Geometry check sheet. Reference: the model listing, model coordinates, mm. Give positions to 0.01 mm unless a question says otherwise; leave off trailing zeros. Loops run counter-clockwise (first coordinate to the right, second up) from the corner with the lowest first, then second, coordinate; pieces in that order, holes last. Notation, with made-up numbers: (24, 54.5) -> (46, 54.5) arc R25 cw to (46, 81.5) -> close; hole circle Ø1 at (50.25, 37.5). An arc over 180 degrees is marked (long way). Answer in a Markdown table with one row per item. Add a question column.
```python
from build123d import *

# Parameters (mm, degrees)
SKETCH1_R                        = 17.5
BOSS_EXTRUDE1_DEPTH              = 12.5
F_1_2_14_NPSM_TAPPED_HOLE1_D     = 18.9738
F_1_2_14_NPSM_TAPPED_HOLE1_DEPTH = 47.24908
F_1_2_14_NPSM_TAPPED_HOLE1_TIP   = 5.700304607
CHAMFER1_SIZE                    = 5
CHAMFER2_SIZE                    = 2
FILLET1_R                        = 1


with BuildPart() as part:
    # Sketch1 → Boss-Extrude1 (new body, symmetric)
    with BuildSketch(Plane.XY):
        Circle(SKETCH1_R)
    extrude(amount=BOSS_EXTRUDE1_DEPTH, both=True)

    # 1/2-14 NPSM Tapped Hole1
    with Locations(Plane.XY.offset(12.5)):
        with Locations((0, 0)):
            Hole(F_1_2_14_NPSM_TAPPED_HOLE1_D / 2, depth=F_1_2_14_NPSM_TAPPED_HOLE1_DEPTH)
            with Locations((0, 0, -(F_1_2_14_NPSM_TAPPED_HOLE1_DEPTH + F_1_2_14_NPSM_TAPPED_HOLE1_TIP / 2))):  # 118° drill point
                Cone(0, F_1_2_14_NPSM_TAPPED_HOLE1_D / 2, F_1_2_14_NPSM_TAPPED_HOLE1_TIP, mode=Mode.SUBTRACT)

    # Chamfer1
    chamfer1_edges = [part.edges().sort_by_distance(p)[0] for p in [
        (-17.5, 0, -12.5),
    ]]
    chamfer(chamfer1_edges, length=CHAMFER1_SIZE)

    # Chamfer2
    chamfer2_edges = [part.edges().sort_by_distance(p)[0] for p in [
        (9.4869, 0, 12.5),
    ]]
    chamfer(chamfer2_edges, length=CHAMFER2_SIZE)

    # Fillet1
    fillet1_edges = [part.edges().sort_by_distance(p)[0] for p in [
        (-17.5, 0, 12.5),
    ]]
    fillet(fillet1_edges, radius=FILLET1_R)


solid = part.part
```
1. Sectioned sample at A-A (y = 0). Enter the section's corners in (x, z).
2. Sectioned sample at C-C (z = 4.5). Enter the section's corners in (x, y).
3. Gauge pin test, flat ends, axial feed: pin 1 Ø15 at (x, y) = (0, 0) entering from -Z; pin 2 Ø10 at (y, z) = (0.5, -7) entering from +X; pin 3 Ø5 at (y, z) = (-10, 5.5) entering from +X; pin 4 Ø3 at (x, y) = (-7, -6.5) entering from +Z. Record the tip position at first contact, or that the pin passes through.
4. Release check for a two-part mould opening along Y. For faces 1 (the face through (-13.887, -10.648, 2.133)), 2 (the face through (6.992, 6.412, -1.161)), 3 (the face through (3.4, 11.2, 12.5)) record: released by +Y, released by -Y, zero draft, split by the parting line, or undercut.
5. Material ranges on L1, parallel to Y at x = 0, z = -6.5; L2, parallel to Z at x = 13.5, y = 0.5; L3, parallel to Y at x = -4, z = 0.75, recorded low to high. Write a range as from..to.
Response:
| question | item | result |
|---|---|---|
| 1 | outline | (-17.5, -7.5) -> (-12.5, -12.5) -> (-9.49, -12.5) -> (-9.49, 10.5) -> (-11.49, 12.5) -> (-16.5, 12.5) arc R1 ccw to (-17.5, 11.5) -> close; (9.49, -12.5) -> (12.5, -12.5) -> (17.5, -7.5) -> (17.5, 11.5) arc R1 ccw to (16.5, 12.5) -> (11.49, 12.5) -> (9.49, 10.5) -> close |
| 2 | outline | circle Ø35 at (0, 0); hole circle Ø18.97 at (0, 0) |
| 3 | pin 1 | passes through |
| 3 | pin 2 | stops at x = 17.5 |
| 3 | pin 3 | stops at x = 15.81 |
| 3 | pin 4 | stops at z = 12.07 |
| 4 | face 1 | split by the parting line |
| 4 | face 2 | undercut |
| 4 | face 3 | zero draft |
| 5 | L1 | y = -17.5..-9.49, 9.49..17.5 |
| 5 | L2 | z = -11.49..12.5 |
| 5 | L3 | y = -17.04..-8.6, 8.6..17.04 |
